Model file for the job. Use its own axes, mm. A direction names the side the tool comes from. Give positions to 0.01 mm unless a question says otherwise; leave off trailing zeros. Order: outer loops, then holes, each group sorted by start corner. A loop starts at its lowest first (then second) coordinate and runs counter-clockwise, first axis right, second up. Notation, with made-up numbers: M -32,9 L 16,9 A21 ccw 16,34 Z; hole C 39,22.25 d6. An arc over 180 degrees is marked long. Return JSON: item names as keys, results as strings. Group by question number.
1. Slice it at C-C on z = 3. List the corners of the cut face in (x, y).
2. 3-axis set-ups, long thin cutter, end or side, ignore diameter. For faces 1 (the face through (0, -22.5, 25)), 2 (the face through (-10, 10, 10)): which of +Z, -Z, +X, -X, +Y, -Y reach the whole face in a straight line?
3. Slice it at A-A on y = 10. List the corners of the cut face in (x, z).
4. Slice it at B-B on x = 0. List the corners of the cut face in (y, z), then the cut area to 3 significant figures.
5. Wall check: probe 1 along Z at (x, y) = (6.5, -12); probe 2 along Z at (x, y) = (1, 3.5); probe 3 along X at (y, z) = (-6, 9). Give the ranges that are in metal, low to high. Write a range as [from, to].
6. Pin check, flat tips, straight feed: pin 1 (4 mm diameter, centred on x = -3.5, y = 15, fed in from -Z); pin 2 (1.5 mm diameter, centred on x = -3.5, z = 0.5, fed in from -Y). Stop position of each tip, or through.
from build123d import *

# Parameters (mm, degrees)
SKETCH1_R           = 12.5
BOSS_EXTRUDE1_DEPTH = 10
SKETCH2_W           = 45
SKETCH2_H           = 45
BOSS_EXTRUDE2_DEPTH = 30
SKETCH4_R           = 2.5
BOSS_EXTRUDE3_DEPTH = 20


with BuildPart() as part:
    # Sketch1 → Boss-Extrude1 (new body)
    with BuildSketch(Plane.XY):
        Circle(SKETCH1_R)
    extrude(amount=BOSS_EXTRUDE1_DEPTH)

    # Sketch2 → Boss-Extrude2 (add)
    with BuildSketch(Plane.XY.offset(10)):
        Rectangle(SKETCH2_W, SKETCH2_H)
    extrude(amount=BOSS_EXTRUDE2_DEPTH)

    # Sketch4 → Boss-Extrude3 (add)
    with BuildSketch(Plane(origin=(0, 0, 0), x_dir=(-1, 0, 0), z_dir=(0, 0, -1))):
        Circle(SKETCH4_R)
    extrude(amount=BOSS_EXTRUDE3_DEPTH)


solid = part.part
Result:
{
 "1": {"outline": "C 0,0 d25"},
 "2": {"face 1": "+Z, -Z, +X, -X, -Y", "face 2": "-Z"},
 "3": {"outline": "M -22.5,10 L -7.5,10 L -7.5,0 L 7.5,0 L 7.5,10 L 22.5,10 L 22.5,40 L -22.5,40 Z"},
 "4": {"outline": "M -22.5,10 L -12.5,10 L -12.5,0 L -2.5,0 L -2.5,-20 L 2.5,-20 L 2.5,0 L 12.5,0 L 12.5,10 L 22.5,10 L 22.5,40 L -22.5,40 Z", "area": "1,700 mm2"},
 "5": {"probe 1": "z = [10, 40]", "probe 2": "z = [0, 40]", "probe 3": "x = [-10.97, 10.97]"},
 "6": {"pin 1": "stops at z = 10", "pin 2": "stops at y = -12.19"}
}
